Part print with two shaded views. Sizes in mm from the minimum x, y, z corner. A direction names the side the tool comes from. Round coordinates to 2 decimals unless told otherwise and drop trailing zeros. Order: outer loops, then holes, each group sorted by start corner. A loop starts at its lowest first (then second) coordinate and runs counter-clockwise, first axis right, second up. Notation, with made-up numbers: M 75,35.25 L 116,35.25 A15 cw 116,50.25 Z; hole C -34.5,68 d8. An arc over 180 degrees is marked long. Answer as a JSON object with one key per item and string values.
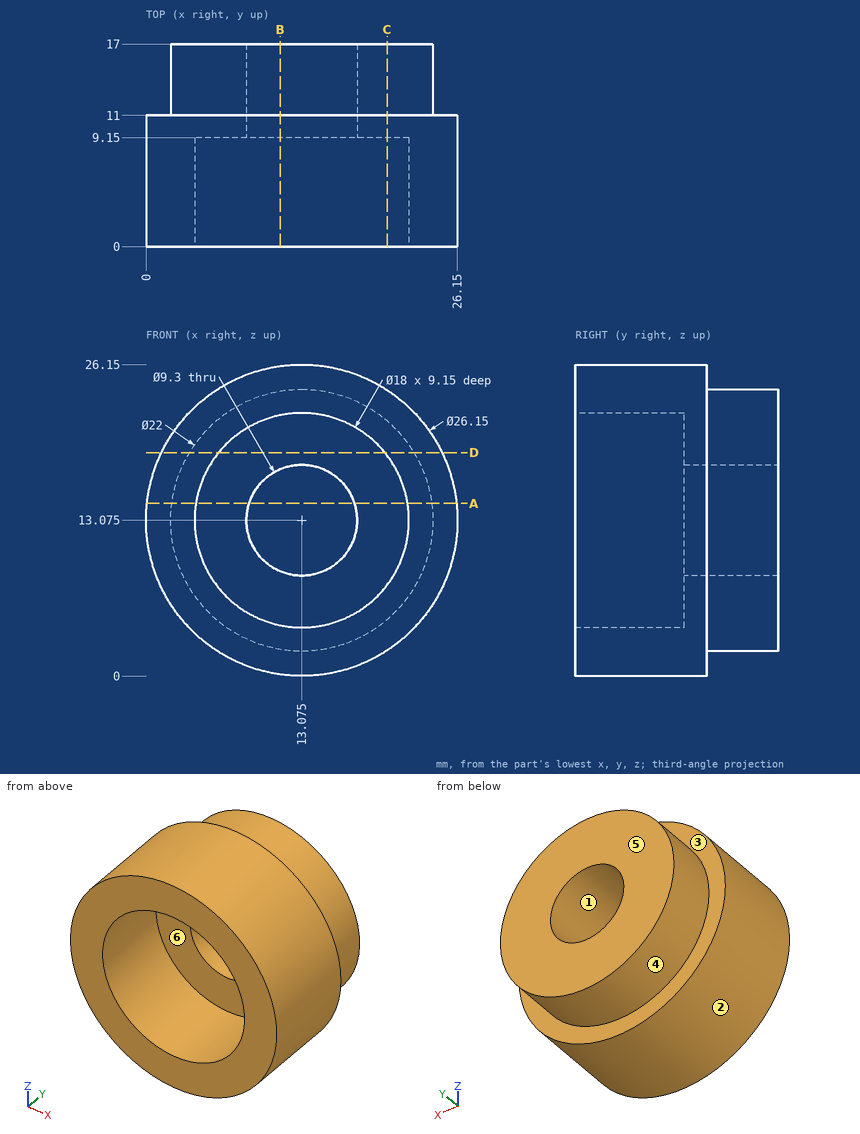
Item 1: Saw through at A-A on z = 14.5. List the corners of the cut face in (x, y).
Worked answers:
{"outline": "M 0.08,0 L 4.19,0 L 4.19,9.15 L 8.65,9.15 L 8.65,17 L 2.17,17 L 2.17,11 L 0.08,11 Z; M 17.5,9.15 L 21.96,9.15 L 21.96,0 L 26.07,0 L 26.07,11 L 23.98,11 L 23.98,17 L 17.5,17 Z"}
Item 2: Wall check: line 1 along Y through (x, z) = (12.25, 5); line 2 along Y through (x, z) = (9.25, 24); line 3 along Z through (x, y) = (19, 3.5). Give the ranges that are in metal, low to high. Write a range as [from, to].
Worked answers:
{"line 1": "y = [9.15, 17]", "line 2": "y = [0, 11]", "line 3": "z = [1.42, 6.3], [19.85, 24.73]"}
Item 3: Drop flat-ended pins along their axis: pin 1 Ø4 at (x, y) = (16.5, 12) entering from -Z; pin 2 Ø1 at (x, y) = (8.5, 12) entering from -Z; pin 3 Ø1.5 at (x, z) = (10, 16) entering from -Y. Give the stop position or say it passes through.
Worked answers:
{"pin 1": "stops at z = 0.11", "pin 2": "stops at z = 2.86", "pin 3": "stops at y = 9.15"}
Item 4: Saw through at C-C on x = 20.25. List the corners of the cut face in (y, z).
Worked answers:
{"outline": "M 0,2.14 L 11,2.14 L 11,4.74 L 17,4.74 L 17,21.41 L 11,21.41 L 11,24.01 L 0,24.01 L 0,18.51 L 9.15,18.51 L 9.15,7.64 L 0,7.64 Z"}
Item 5: Saw through at B-B on x = 11.25. List the corners of the cut face in (y, z).
Worked answers:
{"outline": "M 0,0.13 L 11,0.13 L 11,2.23 L 17,2.23 L 17,8.8 L 9.15,8.8 L 9.15,4.26 L 0,4.26 Z; M 0,21.89 L 9.15,21.89 L 9.15,17.35 L 17,17.35 L 17,23.92 L 11,23.92 L 11,26.02 L 0,26.02 Z"}
Item 6: 3-axis set-ups, long thin cutter, end or side, ignore diameter. For the marked faces 4, 5 and 6: which of +Z, -Z, +X, -X, +Y, -Y reach the whole face in a straight line?
Worked answers:
{"face 4": "+Y", "face 5": "+Z, -Z, +X, -X, +Y", "face 6": "-Y"}
Item 7: Two-plate mould, pull along Z, no slides. Class the marked faces 1, 2 and 3: released by +Z, released by -Z, zero draft, split by the parting line, or undercut.
Worked answers:
{"face 1": "undercut", "face 2": "split by the parting line", "face 3": "zero draft"}
Item 8: Saw through at D-D on z = 18.75. List the corners of the cut face in (x, y).
Worked answers:
{"outline": "M 1.3,0 L 6.09,0 L 6.09,9.15 L 20.06,9.15 L 20.06,0 L 24.85,0 L 24.85,11 L 22.5,11 L 22.5,17 L 3.65,17 L 3.65,11 L 1.3,11 Z"}
